Can you work these out from the model? Positions are in its coordinate system, mm. Face numbers are marked on the shaded views. A direction names the side the tool comes from. Give positions to 0.01 mm unless a question says otherwise; leave off trailing zeros. Write each loop counter-clockwise with the first axis right and the second up, starting at its lowest first coordinate (ties: lowest second). Pieces come first, ordered by that corner, then holes. Notation, with made-up numbers: (69, 65.5) -> (94, 65.5) arc R17 ccw to (94, 97.5) -> close; hole circle Ø2 at (-14.5, 0.25). An arc over 180 degrees is marked (long way). One line per item, written item: value.
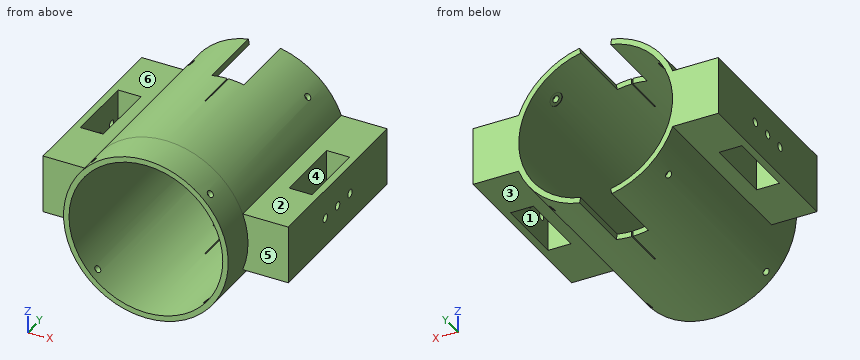
from build123d import *

# Parameters (mm, degrees)
SKETCH1_R                = 33.6
BOSS_EXTRUDE2_DEPTH      = 80
CUT_EXTRUDE3_DEPTH       = 103.805447326
CUT_EXTRUDE3_DEPTH_BACK  = 29.7
CUT_EXTRUDE4_DEPTH       = 103.805447326
CUT_EXTRUDE4_DEPTH_BACK  = 103.805447326
SKETCH7_W                = 0.5
SKETCH7_H                = 18.3
SKETCH9_W                = 10
SKETCH9_H                = 30.5
CUT_EXTRUDE5_DEPTH       = 108.910379482
SKETCH10_R               = 1.75
CUT_EXTRUDE6_DEPTH       = 10
BOSS_EXTRUDE3_REACH      = 120.799
BOSS_EXTRUDE3_END_RADIUS = 33.6
SKETCH11_R               = 3
SKETCH12_R               = 3
CUT_EXTRUDE7_DEPTH       = 10.2
SKETCH13_R               = 1.5
CUT_EXTRUDE9_DEPTH       = 119.798640203
CIRPATTERN1_COUNT        = 4
BOSS_EXTRUDE4_START      = 16
SKETCH14_R               = 36
SKETCH14_R_2             = 33.6
BOSS_EXTRUDE4_DEPTH      = 16
SKETCH17_R               = 1.5
CUT_EXTRUDE10_DEPTH      = 103.805447439
CIRPATTERN2_COUNT        = 4


with BuildPart() as part:
    # Sketch1 → Boss-Extrude2 (new body)
    with BuildSketch(Plane(origin=(0, 0, 0), x_dir=(1, 0, 0), z_dir=(0, 1, 0))):
        with BuildLine():
            ThreePointArc((33.685456803, 12.7), (0, 36), (-33.685456803, 12.7))
            Line((-33.685456803, 12.7), (-53.6, 12.7))
            Line((-53.6, 12.7), (-53.6, -12.7))
            Line((-53.6, -12.7), (-33.685456803, -12.7))
            ThreePointArc((-33.685456803, -12.7), (0, -36), (33.685456803, -12.7))
            Line((33.685456803, -12.7), (53.6, -12.7))
            Line((53.6, -12.7), (53.6, 12.7))
            Line((53.6, 12.7), (33.685456803, 12.7))
        make_face()
        with Locations(Location((0, 0, 0), (0, 0, 270))):
            Circle(SKETCH1_R, mode=Mode.SUBTRACT)
    extrude(amount=BOSS_EXTRUDE2_DEPTH)

    # Sketch6 → Cut-Extrude3 (cut, two sides: drawn at the far end of the back side and taken through both)
    with BuildSketch(Plane(origin=(0, 80, 0), x_dir=(1, 0, 0), z_dir=(0, 1, 0)).offset(-CUT_EXTRUDE3_DEPTH_BACK)):
        with BuildLine():
            Line((-7.023251593, 35.308270095), (-6.55503482, 32.954385422))
            ThreePointArc((-6.55503482, 32.954385422), (0, 33.6), (6.55503482, 32.954385422))
            Line((6.55503482, 32.954385422), (7.023251593, 35.308270095))
            ThreePointArc((7.023251593, 35.308270095), (0, 36), (-7.023251593, 35.308270095))
        make_face()
        with BuildLine():
            Line((-7.023251593, -35.308270095), (-6.55503482, -32.954385422))
            ThreePointArc((-6.55503482, -32.954385422), (0, -33.6), (6.55503482, -32.954385422))
            Line((6.55503482, -32.954385422), (7.023251593, -35.308270095))
            ThreePointArc((7.023251593, -35.308270095), (0, -36), (-7.023251593, -35.308270095))
        make_face()
    extrude(amount=CUT_EXTRUDE3_DEPTH + CUT_EXTRUDE3_DEPTH_BACK, mode=Mode.SUBTRACT)

    # Sketch7 → Cut-Extrude4 (cut, two sides: drawn at the far end of the back side and taken through both)
    with BuildSketch(Plane.XY.offset(-CUT_EXTRUDE4_DEPTH_BACK)):
        with Locations((0, 41.15)):
            Rectangle(SKETCH7_W, SKETCH7_H)
    extrude(amount=CUT_EXTRUDE4_DEPTH + CUT_EXTRUDE4_DEPTH_BACK, mode=Mode.SUBTRACT)

    # Sketch9 → Cut-Extrude5 (cut, through all)
    with BuildSketch(Plane.XY.offset(12.7)):
        with Locations((-45.6, 40)):
            Rectangle(SKETCH9_W, SKETCH9_H)
        with Locations((45.6, 40)):
            Rectangle(SKETCH9_W, SKETCH9_H)
    extrude(amount=-CUT_EXTRUDE5_DEPTH, mode=Mode.SUBTRACT)

    # Sketch10 → Cut-Extrude6 (cut)
    with BuildSketch(Plane.ZY.offset(53.6)):
        with Locations((0, 40)):
            Circle(SKETCH10_R)
        with Locations((0, 50)):
            Circle(SKETCH10_R)
        with Locations((0, 30)):
            Circle(SKETCH10_R)
    cut_extrude6 = extrude(amount=-CUT_EXTRUDE6_DEPTH, mode=Mode.SUBTRACT)

    # Mirror1: Cut-Extrude6 across plane
    add(cut_extrude6.mirror(Plane(origin=(0, 0, 0), x_dir=(0, 0, 1), z_dir=(1, 0, 0))), mode=Mode.SUBTRACT)

    # Boss-Extrude3: up to this cylinder (the profile starts inside it)
    boss_extrude3_end = Plane(origin=(0, 68, 0), z_dir=(0, -1, 0)) * Cylinder(BOSS_EXTRUDE3_END_RADIUS, 309.798, mode=Mode.PRIVATE)
    # Sketch11 → Boss-Extrude3 (add, up to the surface)
    with BuildSketch(Plane(origin=(16.674534964, 0, 16.674534964), x_dir=(0, 1, 0), z_dir=(0.7071067811865488, 0, 0.7071067811865464)), mode=Mode.PRIVATE) as boss_extrude3_sk1:
        with Locations(Location((68, 0, 0), (0, 0, 90))):
            Circle(SKETCH11_R)
    boss_extrude3_tool1 = extrude(boss_extrude3_sk1.sketch, amount=BOSS_EXTRUDE3_REACH, mode=Mode.PRIVATE) & boss_extrude3_end
    boss_extrude3 = boss_extrude3_tool1.solids().sort_by_distance((16.674535, 68, 16.674535))[0]
    add(boss_extrude3)

    # Sketch12 → Cut-Extrude7 (cut)
    with BuildSketch(Plane(origin=(16.674534964, 0, 16.674534964), x_dir=(-0.7071067811865465, 0, 0.7071067811865487), z_dir=(-0.7071067811865487, 0, -0.7071067811865465))):
        with Locations((0, 68)):
            Circle(SKETCH12_R)
    cut_extrude7 = extrude(amount=-CUT_EXTRUDE7_DEPTH, mode=Mode.SUBTRACT)

    # Sketch13 → Cut-Extrude9 (cut, through all)
    with BuildSketch(Plane(origin=(16.674534964, 0, 16.674534964), x_dir=(0, 1, 0), z_dir=(0.7071067811865488, 0, 0.7071067811865464))):
        with Locations(Location((68, 0, 0), (0, 0, 90))):
            Circle(SKETCH13_R)
    cut_extrude9 = extrude(amount=CUT_EXTRUDE9_DEPTH, mode=Mode.SUBTRACT)

    # CirPattern1: Boss-Extrude3, Cut-Extrude7, Cut-Extrude9 ×4 about axis
    cirpattern1_axis = Axis((0, 0, 0), (0, 1, 0))
    add([boss_extrude3.rotate(cirpattern1_axis, i * 360 / CIRPATTERN1_COUNT) for i in range(1, CIRPATTERN1_COUNT)])
    add([cut_extrude7.rotate(cirpattern1_axis, i * 360 / CIRPATTERN1_COUNT) for i in range(1, CIRPATTERN1_COUNT)], mode=Mode.SUBTRACT)
    add([cut_extrude9.rotate(cirpattern1_axis, i * 360 / CIRPATTERN1_COUNT) for i in range(1, CIRPATTERN1_COUNT)], mode=Mode.SUBTRACT)

    # Sketch14 → Boss-Extrude4 (add)
    with BuildSketch(Plane.XZ.offset(BOSS_EXTRUDE4_START)):
        with Locations(Location((0, 0, 0), (0, 0, 270))):
            Circle(SKETCH14_R)
        with Locations(Location((0, 0, 0), (0, 0, 270))):
            Circle(SKETCH14_R_2, mode=Mode.SUBTRACT)
    extrude(amount=-BOSS_EXTRUDE4_DEPTH)

    # Sketch17 → Cut-Extrude10 (cut, through all)
    with BuildSketch(Plane(origin=(0, 0, 0), x_dir=(0, 1, 0), z_dir=(0.7071067811865488, 0, 0.7071067811865464))):
        with Locations(Location((-11, 0, 0), (0, 0, 270))):
            Circle(SKETCH17_R)
    cut_extrude10 = extrude(amount=-CUT_EXTRUDE10_DEPTH, mode=Mode.SUBTRACT)

    # CirPattern2: Cut-Extrude10 ×4 about axis
    cirpattern2_axis = Axis((0, 80, 0), (0, -1, 0))
    for i in range(1, CIRPATTERN2_COUNT):
        add(cut_extrude10.rotate(cirpattern2_axis, i * 360 / CIRPATTERN2_COUNT), mode=Mode.SUBTRACT)


solid = part.part
1) For the marked faces 1, 2 and 3, which set-ups out of +Z, -Z, +X, -X, +Y, -Y let a thin tool reach every point of the face, with its end or its side?
Answer list:
face 1: +Z, -Z
face 2: +Z, +X, +Y, -Y
face 3: -Z, +X, +Y, -Y
2) I need wall thicknesses on L1, parallel to Y at x = 51.8, z = 0; L2, parallel to Z at x = 51, y = 30; L3, parallel to Z at x = 0, y = 8.5. Which ranges of each line are inside material? Lowest first, please.
Answer list:
L1: y = 0 to 28.25, 31.75 to 38.25, 41.75 to 48.25, 51.75 to 80
L2: z = -12.7 to -1.75, 1.75 to 12.7
L3: z = -36 to -33.6, 33.6 to 36
3) If we section it at B-B (z = 6.5): Write out the boundary of the cut face in (x, y).
Answer list:
outline: (-53.6, 0) -> (-35.41, 0) -> (-35.41, -16) -> (-32.97, -16) -> (-32.97, 80) -> (-53.6, 80) -> close; (32.97, -16) -> (35.41, -16) -> (35.41, 0) -> (53.6, 0) -> (53.6, 80) -> (32.97, 80) -> close; hole (-50.6, 24.75) -> (-40.6, 24.75) -> (-40.6, 55.25) -> (-50.6, 55.25) -> close; hole (40.6, 24.75) -> (50.6, 24.75) -> (50.6, 55.25) -> (40.6, 55.25) -> close
4) Will these pins go through, and if not, where does the flat tip stop? pin 1 (4.5 mm diameter, centred on y = 50, z = 0, fed in from +X); pin 2 (2.5 mm diameter, centred on x = 4, z = 34.5, fed in from +Y); pin 3 (22 mm diameter, centred on x = -47, y = 46.5, fed in from +Z); pin 4 (4 mm diameter, centred on x = 41, z = 6, fed in from -Y).
Answer list:
pin 1: stops at x = 53.6
pin 2: stops at y = 50.3
pin 3: stops at z = 12.7
pin 4: stops at y = 0
5) If we section it at C-C (x = 44): Write out the boundary of the cut face in (y, z), and give its area (3 significant figures).
Answer list:
outline: (0, -12.7) -> (24.75, -12.7) -> (24.75, 12.7) -> (0, 12.7) -> close; (55.25, -12.7) -> (80, -12.7) -> (80, 12.7) -> (55.25, 12.7) -> close
area: 1,260 mm^2
6) We'd pull the mould along Y, two halves only. Please class the marked faces 4, 5 and 6: released by +Y, released by -Y, zero draft, split by the parting line, or undercut.
Answer list:
face 4: undercut
face 5: released by -Y
face 6: zero draft
7) If we section it at A-A (y = 30): Write out the boundary of the cut face in (x, z).
Answer list:
outline: (-53.6, -12.7) -> (-50.6, -12.7) -> (-50.6, -1.75) -> (-53.6, -1.75) -> close; (-53.6, 1.75) -> (-50.6, 1.75) -> (-50.6, 12.7) -> (-53.6, 12.7) -> close; (-40.6, -12.7) -> (-33.69, -12.7) arc R36 ccw to (33.69, -12.7) -> (40.6, -12.7) -> (40.6, 12.7) -> (33.69, 12.7) arc R36 ccw to (-33.69, 12.7) -> (-40.6, 12.7) -> close; (50.6, -12.7) -> (53.6, -12.7) -> (53.6, -1.75) -> (50.6, -1.75) -> close; (50.6, 1.75) -> (53.6, 1.75) -> (53.6, 12.7) -> (50.6, 12.7) -> close; hole circle Ø67.2 at (0, 0)
